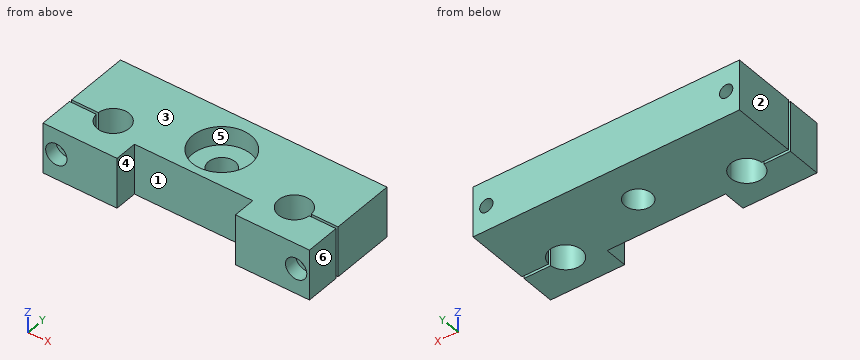
```python
from build123d import *

# Parameters (mm, degrees)
F0_R     = 11
F1_DEPTH = 19
F0_R_2   = 5
F2_DEPTH = 12
F3_R     = 2.5
F4_DEPTH = 38.001
F3_R_2   = 4
F5_DEPTH = 5


with BuildPart() as f1:
    # F0 (on Top) → F1 (new body)
    with BuildSketch(Plane.XY):
        with BuildLine():
            Line((9.388096, -2.975142), (-90.611904, -2.975142))
            Line((-90.611904, -2.975142), (-90.611904, -26.975142))
            Line((-90.611904, -26.975142), (-80.591034, -26.975142))
            ThreePointArc((-80.591034, -26.975142), (-74.361686, -21.480362), (-68.611904, -27.475142))
            ThreePointArc((-68.611904, -27.475142), (-74.361686, -33.469923), (-80.591034, -27.975142))
            Line((-80.591034, -27.975142), (-90.611904, -27.975142))
            Line((-90.611904, -27.975142), (-90.611904, -40.975142))
            Line((-90.611904, -40.975142), (-62.83059, -40.975142))
            Line((-62.83059, -40.975142), (-62.83059, -32.448158))
            Line((-62.83059, -32.448158), (-18.393222, -32.448158))
            Line((-18.393222, -32.448158), (-18.393222, -40.975142))
            Line((-18.393222, -40.975142), (9.388096, -40.975142))
            Line((9.388096, -40.975142), (9.388096, -27.975142))
            Line((9.388096, -27.975142), (-0.632774, -27.975142))
            ThreePointArc((-0.632774, -27.975142), (-12.611904, -27.475142), (-0.632774, -26.975142))
            Line((-0.632774, -26.975142), (9.388096, -26.975142))
            Line((9.388096, -26.975142), (9.388096, -2.975142))
        make_face()
        with Locations((-40.611904, -18.648577)):
            Circle(F0_R, mode=Mode.SUBTRACT)
    extrude(amount=F1_DEPTH)

    # F0 (on Top) → F2 (join)
    with BuildSketch(Plane.XY):
        with Locations((-40.611904, -18.648577)):
            Circle(F0_R)
        with Locations((-40.611904, -18.648577)):
            Circle(F0_R_2, mode=Mode.SUBTRACT)
    extrude(amount=F2_DEPTH)

    # F3 (on face) → F4 (cut, through all)
    with BuildSketch(Plane.XZ.offset(40.975142)):
        with Locations((-85.611904, 9.5)):
            Circle(F3_R)
        with Locations((4.388096, 9.5)):
            Circle(F3_R)
    extrude(amount=-F4_DEPTH, mode=Mode.SUBTRACT)

    # F3 (on face) → F5 (cut)
    with BuildSketch(Plane.XZ.offset(40.975142)):
        with Locations((-85.611904, 9.5)):
            Circle(F3_R_2)
        with Locations((-85.611904, 9.5)):
            Circle(F3_R, mode=Mode.SUBTRACT)
        with Locations((4.388096, 9.5)):
            Circle(F3_R_2)
        with Locations((4.388096, 9.5)):
            Circle(F3_R, mode=Mode.SUBTRACT)
    extrude(amount=-F5_DEPTH, mode=Mode.SUBTRACT)


solid = f1.part
```
Model file for the job. Use its own axes, mm. Face numbers are marked on the shaded views. A direction names the side the tool comes from. Coordinates: 2 decimals unless noted, no trailing zeros. Order: outer loops, then holes, each group sorted by start corner. A loop starts at its lowest first (then second) coordinate and runs counter-clockwise, first axis right, second up. Notation, with made-up numbers: (-36, 71.5) - (18, 71.5) arc R20 ccw to (18, 109.5) - close; hole circle Ø7 at (55, -1). An arc over 180 degrees is marked (long way). Return JSON: item names as keys, results as strings. Group by question number.
1) Tool access for the marked faces 4, 5 and 6: list every direction of +Z, -Z, +X, -X, +Y, -Y with a clear straight run to the whole face (end or side of a thin tool).
2) Probe line 1 (Y direction, x = -74.5, z = 10.5); line 2 (X direction, y = -38.5, z = 16.5); line 3 (X direction, y = -30, z = 7.5). List the from-to ranges inside material, lowest first. Write a range as from..to.
3) Saw through at D-D, the plane z = 9.5. Count the separate pieces of the cut face and the enclosed holes in it, plus the area to 3 significant figures.
4) Saw through at A-A, the plane y = -37. Write the cut outline in (x, z).
5) Flat gauge pins, fed straight in: P1, Ø6.5, axis at x = 4.39, z = 9.5, coming from the -Y side; P2, Ø4, axis at x = -44.5, y = -23, coming from the +Z side; P3, Ø5.5, axis at x = -41, z = 9.5, coming from the -Y side. Where does each tip first touch, or does it go through?
6) Saw through at C-C, the plane y = -5.5. Write the cut outline in (x, z).
7) Saw through at B-B, the plane x = -71. Write the cut outline in (y, z), plus the area to 3 significant figures.
8) Mould opens along X. For the marked faces 1, 2 and 3 say: released by +X, released by -X, zero draft, split by the parting line, or undercut.
Values found:
{
 "1": {"face 4": "+Z, -Z, -Y", "face 5": "+Z", "face 6": "+Z, -Z, +X, +Y, -Y"},
 "2": {"line 1": "y = -40.98..-33.47, -21.48..-2.98", "line 2": "x = -90.61..-62.83, -18.39..9.39", "line 3": "x = -90.61..-87.11, -84.11..-80.05, -69.17..-12.05, -1.17..2.89, 5.89..9.39"},
 "3": {"separate pieces": "5", "enclosed holes": "1", "area": "2,700 mm²"},
 "4": {"outline": "(-90.61, 0) - (-62.83, 0) - (-62.83, 19) - (-90.61, 19) - close; (-18.39, 0) - (9.39, 0) - (9.39, 19) - (-18.39, 19) - close; hole circle Ø8 at (-85.61, 9.5); hole circle Ø8 at (4.39, 9.5)"},
 "5": {"P1": "stops at y = -35.98", "P2": "stops at z = 12", "P3": "stops at y = -32.45"},
 "6": {"outline": "(-90.61, 0) - (9.39, 0) - (9.39, 19) - (-90.61, 19) - close; hole circle Ø5 at (-85.61, 9.5); hole circle Ø5 at (4.39, 9.5)"},
 "7": {"outline": "(-40.98, 0) - (-32.27, 0) - (-32.27, 19) - (-40.98, 19) - close; (-22.68, 0) - (-2.98, 0) - (-2.98, 19) - (-22.68, 19) - close", "area": "540 mm²"},
 "8": {"face 1": "undercut", "face 2": "released by -X", "face 3": "zero draft"}
}
